from build123d import *


with BuildPart() as part:
    # Esquisse1 → Base-Révol.-Mince (revolve)
    with BuildSketch(Plane.XY, mode=Mode.PRIVATE) as base_r_vol_mince_sk:
        with BuildLine():
            Line((0, 37.5), (0, 29.5))
            ThreePointArc((0, 29.5), (0.732233047, 27.732233047), (2.5, 27))
            Line((2.5, 27), (7, 27))
            Line((7, 27), (7, 29))
            Line((7, 29), (2.5, 29))
            ThreePointArc((2.5, 29), (2.146446609, 29.146446609), (2, 29.5))
            Line((2, 29.5), (2, 37.5))
            Line((2, 37.5), (0, 37.5))
        make_face()
    revolve(base_r_vol_mince_sk.sketch.rotate(Axis((0, 0, 0), (1, 0, 0)), 90), axis=Axis((0, 0, 0), (1, 0, 0)))


solid = part.part
Geometry: final body of the model. Coordinates: model frame, mm. A direction names the side the tool comes from. Give positions to 0.01 mm unless a question says otherwise; leave off trailing zeros. Write each loop counter-clockwise with the first axis right and the second up, starting at its lowest first coordinate (ties: lowest second). Pieces come first, ordered by that corner, then holes.
(1) Cut plane A-A, the plane z = 0. Return loops of the section in (x, y).
(2) First-contact query: P1, Ø2, axis at x = 2.5, y = -15, coming from the -Z side; P2, Ø10, axis at y = 0, z = 26.5, coming from the -X side; P3, Ø1, axis at x = 5.5, y = -20.5, coming from the +Z side. Flat tips, straight axial feed; report the tip coordinate or a pass-through.
(3) Cut plane C-C, the plane x = 4. Return loops of the section in (y, z), then the cut area to 3 significant figures.
(4) Mould query, pull axis Z, two halves, no side actions, for faces 1 (the cylindrical face through (4.78, 26.36, -5.85)), 2 (the flat face through (7, 8, -26)), 3 (the cylindrical face through (4.72, 25.73, 13.38)). Classes: released by +Z, released by -Z, zero draft, split by the parting line, or undercut.
(5) Access query for faces 4 (the flat face through (2, 25, -16)), 5 (the cylindrical face through (0.99, 33.27, 17.3)). Directions: +Z, -Z, +X, -X, +Y, -Y. A direction counts if a zero-diameter tool reaches every point of the face in a straight line with its end or side. Return the directions, or none.
(6) Ray query, line 1 (Y direction, x = 5.2, z = 0); line 2 (Z direction, x = 6.5, y = 14.5); line 3 (Z direction, x = 2.75, y = -23). Return the intervals inside material, ascending.
Values follow:
1. outline: (0, -37.5) - (2, -37.5) - (2, -29.5) arc R0.5 cw to (2.5, -29) - (7, -29) - (7, -27) - (2.5, -27) arc R2.5 ccw to (0, -29.5) - close; (0, 29.5) arc R2.5 ccw to (2.5, 27) - (7, 27) - (7, 29) - (2.5, 29) arc R0.5 cw to (2, 29.5) - (2, 37.5) - (0, 37.5) - close
2. P1: stops at z = -34.73
2. P2: stops at x = 0
2. P3: stops at z = 21
3. outline: circle Ø58 at (0, 0); hole circle Ø54 at (0, 0)
3. area: 352 mm2
4. face 1: undercut
4. face 2: zero draft
4. face 3: split by the parting line
5. face 4: +X
5. face 5: +X, -X
6. line 1: y = -29 to -27, 27 to 29
6. line 2: z = -25.11 to -22.78, 22.78 to 25.11
6. line 3: z = -17.66 to -14.14, 14.14 to 17.66
